```python
from build123d import *

# Parameters (mm, degrees)
F1_DEPTH = 63.5
F0_W     = 25.4
F0_H     = 19.05
F2_DEPTH = 25.4
F3_DEPTH = 7.9375
F5_R     = 6.35
F6_D     = 21.03374
F6_DEPTH = 63.501


with BuildPart() as f1:
    # F0 (on Front) → F1 (new body, symmetric)
    with BuildSketch(Plane.XZ):
        Polygon((-41.275, -9.525), (41.275, -9.525), (41.275, 9.525), (22.225, 9.525), (-41.275, 9.525), align=None)
    extrude(amount=F1_DEPTH, both=True)

    # F0 (on Front) → F2 (join, symmetric)
    with BuildSketch(Plane.XZ):
        with BuildLine():
            Line((22.225, 9.525), (41.275, 9.525))
            Line((41.275, 9.525), (41.275, 27.0002))
            ThreePointArc((41.275, 27.0002), (45.9246798487, 38.2255201513), (57.15, 42.8752))
            Line((57.15, 42.8752), (60.325, 42.8752))
            Line((60.325, 42.8752), (60.325, 61.9252))
            Line((60.325, 61.9252), (57.15, 61.9252))
            ThreePointArc((57.15, 61.9252), (32.4542956671, 51.6959043329), (22.225, 27.0002))
            Line((22.225, 27.0002), (22.225, 9.525))
        make_face()
        with Locations((73.025, 52.4002)):
            Rectangle(F0_W, F0_H)
    extrude(amount=F2_DEPTH, both=True)

    # F0 (on Front) → F3 (join, symmetric)
    with BuildSketch(Plane.XZ):
        with BuildLine():
            add(Edge.make_bspline(
                [(-41.275, 9.525), (-38.1687022746, 30.0928875804), (14.3155772239, 64.0365257859), (57.15, 61.9252)],
                knots=[0, 0, 0, 0, 111.5045361635, 111.5045361635, 111.5045361635, 111.5045361635], degree=3))
            Line((-41.275, 9.525), (22.225, 9.525))
            Line((22.225, 9.525), (22.225, 27.0002))
            ThreePointArc((22.225, 27.0002), (32.4542956671, 51.6959043329), (57.15, 61.9252))
        make_face()
    extrude(amount=F3_DEPTH, both=True)

    # F0 (on Front) → F4 (revolve)
    with BuildSketch(Plane.XZ):
        Polygon((85.725, 66.675), (85.725, 61.9252), (85.725, 42.8752), (85.725, 38.1), (111.125, 38.1), (111.125, 66.675), align=None)
    revolve(axis=Axis((85.725, 0, 52.3875), (0, 0, 1)))

    # F5
    f5_edges = [f1.edges().sort_by_distance(p)[0] for p in [
        (-41.275, -63.5, 0),
        (41.275, -63.5, 0),
        (41.275, 63.5, 0),
        (-41.275, 63.5, 0),
    ]]
    fillet(f5_edges, radius=F5_R)

    # F6 (through all, one way)
    with BuildSketch(Plane.XZ):
        with Locations((85.725, 66.675)):
            Circle(F6_D / 2)
    extrude(amount=-F6_DEPTH, mode=Mode.SUBTRACT)


solid = f1.part
```
CAD build for the part. Positions are in the model's coordinates, mm. A direction names the side the tool comes from. Coordinates: 2 decimals unless noted, no trailing zeros. Write each loop counter-clockwise with the first axis right and the second up, starting at its lowest first coordinate (ties: lowest second). Pieces come first, ordered by that corner, then holes.
(1) Drill centre lines: probe 1 along Z at (x, y) = (-29, -41) (3 decimals); probe 2 along Y at (x, z) = (59, 60.5); probe 3 along Y at (x, z) = (-11, 22). Where is each one in solid material? Low to high.
(2) Cut at A-A, the plane z = 0. List the corners of the cut face in (x, y) (3 decimals).
(3) Cut at C-C, the plane y = -11. List the corners of the cut face in (x, z) (3 decimals), and give its area (3 significant figures).
(4) Cut at B-B, the plane y = -52.5. List the corners of the cut face in (x, z) (3 decimals), and give its area (3 significant figures).
(5) Flat gauge pins, fed straight in: pin 1 (14.5 mm diameter, centred on x = 76, y = 8, fed in from -Z); pin 2 (3 mm diameter, centred on x = 85.5, z = 59, fed in from +Y); pin 3 (8.5 mm diameter, centred on y = -18.5, z = 14, fed in from -X) (3 decimals). Where does each tip first touch, or does it go through?
(6) 3-axis set-ups, long thin cutter, end or side, ignore diameter. For faces 1 (the face through (86, 0, 38.1)), 2 (the face through (32.73, -16.79, 51.97)): which of +Z, -Z, +X, -X, +Y, -Y reach the whole face in a straight line?
Geometry says:
1. probe 1: z = -9.525 to 9.525
1. probe 2: y = -25.4 to 25.4
1. probe 3: y = -7.94 to 7.94
2. outline: (-41.275, -57.15) arc R6.35 ccw to (-34.925, -63.5) - (34.925, -63.5) arc R6.35 ccw to (41.275, -57.15) - (41.275, 57.15) arc R6.35 ccw to (34.925, 63.5) - (-34.925, 63.5) arc R6.35 ccw to (-41.275, 57.15) - close
3. outline: (-41.275, -9.525) - (41.275, -9.525) - (41.275, 27) arc R15.875 cw to (57.15, 42.875) - (62.83, 42.875) - (62.83, 38.1) - (108.62, 38.1) - (108.62, 66.675) - (62.83, 66.675) - (62.83, 61.925) - (57.15, 61.925) arc R34.925 ccw to (22.225, 27) - (22.225, 9.525) - (-41.275, 9.525) - close
3. area: 4,080 mm2
4. outline: (-41.275, -9.525) - (41.275, -9.525) - (41.275, 9.525) - (-41.275, 9.525) - close
4. area: 1,570 mm2
5. pin 1: stops at z = 38.1
5. pin 2: stops at y = 0
5. pin 3: stops at x = 22.225
6. face 1: -Z, +X, +Y, -Y
6. face 2: +Z, -X, -Y
